Verification items for this drawing (mm, ordinates from the low corner). A direction names the side the tool comes from. Give positions to 0.01 mm unless a question says otherwise; leave off trailing zeros. Write each loop counter-clockwise with the first axis right and the second up, starting at its lowest first coordinate (ties: lowest second). Pieces come first, ordered by that corner, then holes. Notation, with made-up numbers: (47.25, -36.75) -> (69.25, -36.75) arc R15 cw to (69.25, -15.75) -> close; hole circle Ø5 at (-14.5, -37.75). An arc over 180 degrees is marked (long way). Answer as a JSON object with one key per item and string values.
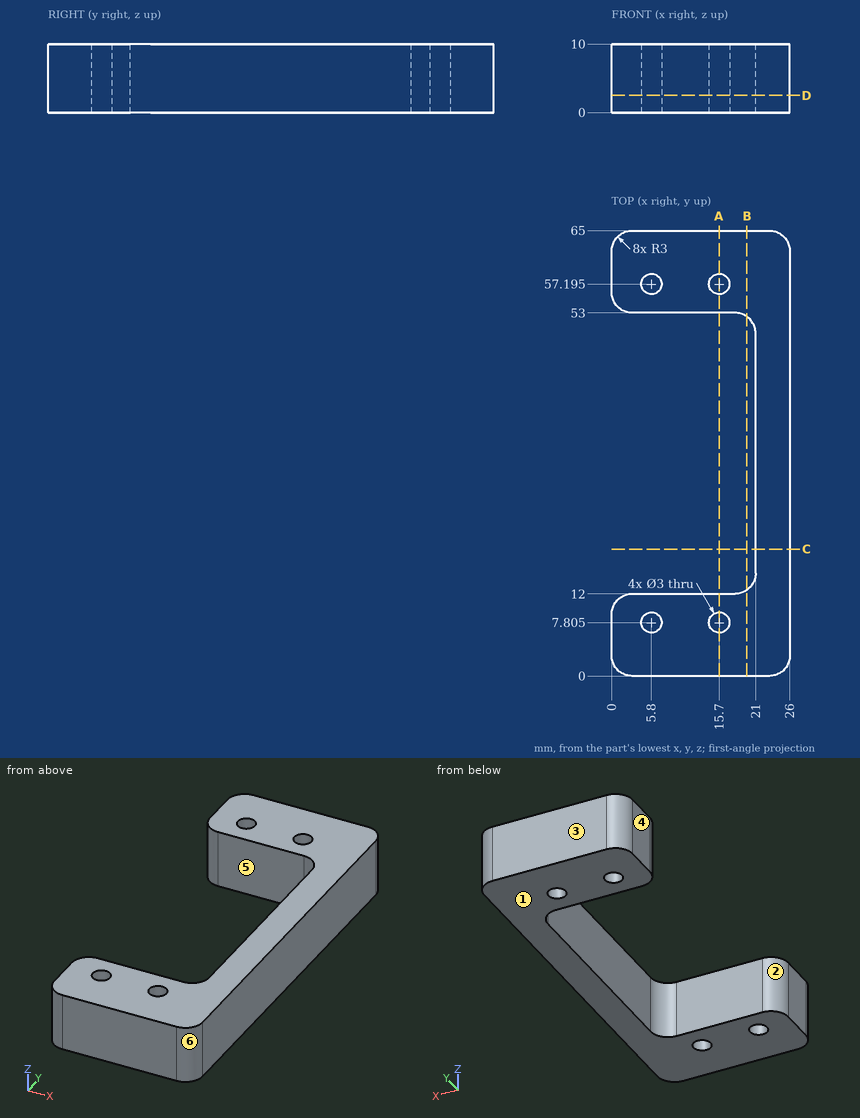
1. Scan lines: L1, parallel to Y at x = 15.7, z = 5 (3 decimals); L2, parallel to Y at x = 9.5, z = 2; L3, parallel to Y at x = 6.5, z = 5.5. Record each from-to range of solid material in increasing order. Write a range as [from, to].
Determined:
{"L1": "[0, 6.305], [9.305, 12], [53, 55.695], [58.695, 65]", "L2": "[0, 12], [53, 65]", "L3": "[0, 6.48], [9.13, 12], [53, 55.87], [58.52, 65]"}
2. Sectioned sample at B-B, the plane x = 19.75. Enter the section's corners in (y, z), plus the area to 3 significant figures.
Determined:
{"outline": "(0, 0) -> (12.56, 0) -> (12.56, 10) -> (0, 10) -> close; (52.44, 0) -> (65, 0) -> (65, 10) -> (52.44, 10) -> close", "area": "251 mm^2"}
3. Mould release check, pull along Y, two halves, no side actions. Record for the marked faces 3, 4, 5 and 6: released by +Y, released by -Y, zero draft, split by the parting line, or undercut.
Determined:
{"face 3": "released by +Y", "face 4": "zero draft", "face 5": "undercut", "face 6": "released by -Y"}
4. Sectioned sample at D-D, the plane z = 2.5. Enter the section's corners in (x, y) (3 decimals).
Determined:
{"outline": "(0, 3) arc R3 ccw to (3, 0) -> (23, 0) arc R3 ccw to (26, 3) -> (26, 62) arc R3 ccw to (23, 65) -> (3, 65) arc R3 ccw to (0, 62) -> (0, 56) arc R3 ccw to (3, 53) -> (18, 53) arc R3 cw to (21, 50) -> (21, 15) arc R3 cw to (18, 12) -> (3, 12) arc R3 ccw to (0, 9) -> close; hole circle Ø3 at (5.8, 7.805); hole circle Ø3 at (5.8, 57.195); hole circle Ø3 at (15.7, 7.805); hole circle Ø3 at (15.7, 57.195)"}
5. Sectioned sample at A-A, the plane x = 15.7. Enter the section's corners in (y, z) (3 decimals).
Determined:
{"outline": "(0, 0) -> (6.305, 0) -> (6.305, 10) -> (0, 10) -> close; (9.305, 0) -> (12, 0) -> (12, 10) -> (9.305, 10) -> close; (53, 0) -> (55.695, 0) -> (55.695, 10) -> (53, 10) -> close; (58.695, 0) -> (65, 0) -> (65, 10) -> (58.695, 10) -> close"}
6. Access from +Z, -Z, +X, -X, +Y, -Y to the whole of each face (thin tool, end or side, straight path). Record for the marked faces 1 and 2.
Determined:
{"face 1": "-Z, +X, -X, +Y, -Y", "face 2": "+Z, -Z, -X"}
7. Sectioned sample at C-C, the plane y = 18.5. Enter the section's corners in (x, z), plus the area to 3 significant figures.
Determined:
{"outline": "(21, 0) -> (26, 0) -> (26, 10) -> (21, 10) -> close", "area": "50.0 mm^2"}
8. Go/stop test with flat-tipped pins: P1, Ø5, axis at x = 5.8, y = 57.195, coming from the -Z side; P2, Ø5, axis at y = 40, z = 7.5, coming from the -X side. Record where each tip stops, or that it passes through.
Determined:
{"P1": "z = 0", "P2": "x = 21"}
